Could you check a few things on this model? Use its own coordinates, in mm. Face numbers are marked on the shaded views. Give positions to 0.01 mm unless a question says otherwise; leave off trailing zeros. Loops run counter-clockwise (first coordinate to the right, second up) from the corner with the lowest first, then second, coordinate; pieces in that order, holes last.
1. Imagine slicing it at A-A (y = 7.25). List the corners of the cut face in (x, z) for me, plus the area to 3 significant figures.
2. I need wall thicknesses on line 1 along X through (y, z) = (7.5, 15.5); line 2 along Z through (x, y) = (4, 2). Which ranges of each line are inside material? Lowest first, please.
3. Imagine slicing it at C-C (x = 15). Count the separate pieces of the cut face and the enclosed holes in it, plus the area to 3 significant figures.
4. Imagine slicing it at B-B (z = 2). List the corners of the cut face in (x, y) for me.
5. Thinking about a two-plate mould opening in Z: for the marked faces 1 and 2, which applies, +Z half, -Z half, draft (parallel to the pull), parting line (faces both ways), or undercut?
6. For P1, Ø1.1, axis at x = -2, z = 17.5, coming from the +Y side; P2, Ø1, axis at y = 9.5, z = -12, coming from the +X side; P3, Ø1.5, axis at x = 13, y = 4.5, coming from the -Z side; P4, Ø3, axis at x = -15.5, z = -15.5, coming from the +Y side, each with a flat end and sliding along its axis, tell me the tip position at first contact or that it passes through.
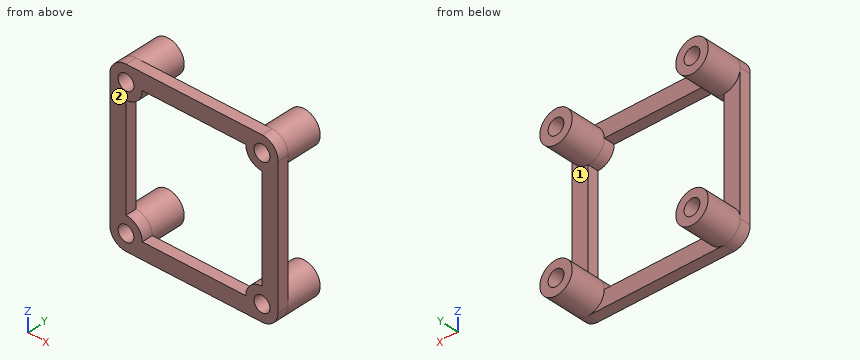
```python
from build123d import *

# Parameters (mm, degrees)
SKETCH_1_R      = 1.8
EXTRUDE_1_DEPTH = 2.5
SKETCH_2_R      = 3.7
SKETCH_2_R_2    = 1.8
EXTRUDE_2_DEPTH = 8


with BuildPart() as part:
    # 草图1 → 凸台-拉伸1 (new body)
    with BuildSketch(Plane(origin=(0, 0, 0), x_dir=(1, 0, 0), z_dir=(0, 1, 0))):
        with BuildLine():
            Line((-19.2, 15.5), (-19.2, -15.5))
            ThreePointArc((-19.2, -15.5), (-18.11629509, -18.11629509), (-15.5, -19.2))
            Line((-15.5, -19.2), (15.5, -19.2))
            ThreePointArc((15.5, -19.2), (18.11629509, -18.11629509), (19.2, -15.5))
            Line((19.2, -15.5), (19.2, 15.5))
            ThreePointArc((19.2, 15.5), (18.11629509, 18.11629509), (15.5, 19.2))
            Line((15.5, 19.2), (-15.5, 19.2))
            ThreePointArc((-15.5, 19.2), (-18.11629509, 18.11629509), (-19.2, 15.5))
        make_face()
        with Locations((-15.5, 15.5)):
            Circle(SKETCH_1_R, mode=Mode.SUBTRACT)
        with Locations((15.5, 15.5)):
            Circle(SKETCH_1_R, mode=Mode.SUBTRACT)
        with Locations((-15.5, -15.5)):
            Circle(SKETCH_1_R, mode=Mode.SUBTRACT)
        with Locations((15.5, -15.5)):
            Circle(SKETCH_1_R, mode=Mode.SUBTRACT)
        with BuildLine():
            Line((-11.8, 15.5), (11.8, 15.5))
            ThreePointArc((11.8, 15.5), (12.88370491, 12.88370491), (15.5, 11.8))
            Line((15.5, 11.8), (15.5, -11.8))
            ThreePointArc((15.5, -11.8), (12.88370491, -12.88370491), (11.8, -15.5))
            Line((11.8, -15.5), (-11.8, -15.5))
            ThreePointArc((-11.8, -15.5), (-12.88370491, -12.88370491), (-15.5, -11.8))
            Line((-15.5, -11.8), (-15.5, 11.8))
            ThreePointArc((-15.5, 11.8), (-12.88370491, 12.88370491), (-11.8, 15.5))
        make_face(mode=Mode.SUBTRACT)
    extrude(amount=EXTRUDE_1_DEPTH)

    # 草图2 → 凸台-拉伸2 (add)
    with BuildSketch(Plane(origin=(0, 2.5, 0), x_dir=(1, 0, 0), z_dir=(0, 1, 0))):
        with Locations((-15.5, 15.5)):
            Circle(SKETCH_2_R)
        with Locations((-15.5, 15.5)):
            Circle(SKETCH_2_R_2, mode=Mode.SUBTRACT)
        with Locations((15.5, 15.5)):
            Circle(SKETCH_2_R)
        with Locations((15.5, 15.5)):
            Circle(SKETCH_2_R_2, mode=Mode.SUBTRACT)
        with Locations((15.5, -15.5)):
            Circle(SKETCH_2_R)
        with Locations((15.5, -15.5)):
            Circle(SKETCH_2_R_2, mode=Mode.SUBTRACT)
        with Locations((-15.5, -15.5)):
            Circle(SKETCH_2_R)
        with Locations((-15.5, -15.5)):
            Circle(SKETCH_2_R_2, mode=Mode.SUBTRACT)
    extrude(amount=EXTRUDE_2_DEPTH)


solid = part.part
```
Derived:
1. outline: circle Ø7.4 at (-15.5, -15.5); circle Ø7.4 at (-15.5, 15.5); circle Ø7.4 at (15.5, -15.5); circle Ø7.4 at (15.5, 15.5); hole circle Ø3.6 at (-15.5, -15.5); hole circle Ø3.6 at (-15.5, 15.5); hole circle Ø3.6 at (15.5, -15.5); hole circle Ø3.6 at (15.5, 15.5)
1. area: 131 mm2
2. line 1: x = -19.2 to -17.3, -13.7 to -11.8, 11.8 to 13.7, 17.3 to 19.2
2. line 2: z = -19.2 to -15.5, 15.5 to 19.2
3. separate pieces: 4
3. enclosed holes: 0
3. area: 81.5 mm2
4. outline: (-19.2, 0) - (-15.5, 0) - (-15.5, 2.5) - (-19.2, 2.5) - close; (15.5, 0) - (19.2, 0) - (19.2, 2.5) - (15.5, 2.5) - close
5. face 1: undercut
5. face 2: draft
6. P1: stops at y = 2.5
6. P2: stops at x = 17.67
6. P3: stops at z = -18.76
6. P4: passes through
